from build123d import *

# Parameters (mm, degrees)
CYLINDER072_R     = 1.3
CYLINDER072_DEPTH = 331
CYLINDER061_R     = 1.3
CYLINDER061_DEPTH = 331
CYLINDER054_W     = 105
CYLINDER054_H     = 10
CYLINDER054_ANGLE = 180
CYLINDER053_W     = 115
CYLINDER053_H     = 10
CYLINDER053_ANGLE = 180


with BuildPart() as cilindro072:
    # Cylinder072 → Cylinder072 (new body)
    with BuildSketch(Plane(origin=(5, 224, 178), x_dir=(0, 0, -1), z_dir=(1, 0, 0))):
        Circle(CYLINDER072_R)
    extrude(amount=CYLINDER072_DEPTH)


with BuildPart() as cilindro061:
    # Cylinder061 → Cylinder061 (new body)
    with BuildSketch(Plane(origin=(5, 6, 178), x_dir=(0, 0, -1), z_dir=(1, 0, 0))):
        Circle(CYLINDER061_R)
    extrude(amount=CYLINDER061_DEPTH)


with BuildPart() as cilindro054:
    # Cylinder054 → Cylinder054 (revolve)
    with BuildSketch(Plane(origin=(-3, 115, 171), x_dir=(0, -1, 0), z_dir=(0, 0, -1))):
        with Locations((52.5, 5)):
            Rectangle(CYLINDER054_W, CYLINDER054_H)
    revolve(axis=Axis((-3, 115, 171), (-1, 0, 0)), revolution_arc=CYLINDER054_ANGLE)


with BuildPart() as cut081:
    # Cylinder053 → Cylinder053 (revolve)
    with BuildSketch(Plane(origin=(-3, 115, 171), x_dir=(0, -1, 0), z_dir=(0, 0, -1))):
        with Locations((57.5, 5)):
            Rectangle(CYLINDER053_W, CYLINDER053_H)
    revolve(axis=Axis((-3, 115, 171), (-1, 0, 0)), revolution_arc=CYLINDER053_ANGLE)

    # Cut067: cut Cilindro054
    add(cilindro054.part, mode=Mode.SUBTRACT)


with BuildPart() as cut081_1:
    # Cut067 placement: moved
    add(cut081.part.moved(Location((343, 0, -9))))

    # Cut072: cut Cilindro061
    add(cilindro061.part, mode=Mode.SUBTRACT)

    # Cut081: cut Cilindro072
    add(cilindro072.part, mode=Mode.SUBTRACT)


solid = cut081_1.part
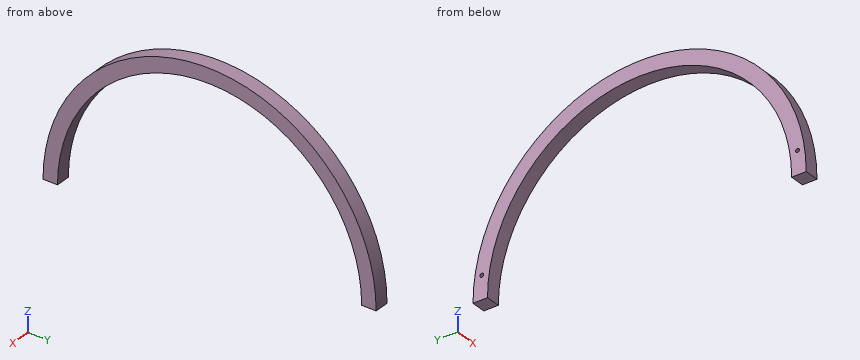
Design review of the part built by this model. Coordinates are the model's own, in mm. Give positions to 0.01 mm unless a question says otherwise; leave off trailing zeros. Order: outer loops, then holes, each group sorted by start corner. A loop starts at its lowest first (then second) coordinate and runs counter-clockwise, first axis right, second up. Notation, with made-up numbers: (25, 81) - (30, 81) arc R14 cw to (30, 105) - close; hole circle Ø6 at (85, -39). An arc over 180 degrees is marked (long way). Write item = value, one per line. Start each with the question number.
Q1. To check wall thickness, follow L1, parallel to Y at x = 333.25, z = 178; L2, parallel to Y at x = 338.5, z = 240; L3, parallel to Y at x = 337, z = 238. State the ranges of each line that lie inside material, in increasing order. Write a range as from..to.
Q2. We need section C-C on y = 115. State the section outline as (x, z) points.
Q3. We need section A-A on z = 195. State the section outline as (x, y) points, plus the area to 3 significant figures.
Q4. Clearance check with flat-ended pins moving along their axes: pin 1 Ø3 at (x, y) = (336.5, 56) entering from +Z; pin 2 Ø2 at (x, z) = (338, 196) entering from -Y; pin 3 Ø3.5 at (y, z) = (6, 178) entering from -X; pin 4 Ø4 at (x, y) = (331.5, 101) entering from +Z. State where each tip first meets the part, or that it passes through.
Q5. We need section B-B on x = 334.5. State the section outline as (y, z) points, plus the area to 3 significant figures.
Q6. We need section D-D on z = 242.5. State the section outline as (x, y) points.
Working result:
q1.L1 = 1.12..4.7, 7.3..11.23, 218.77..222.7, 225.3..228.88
q1.L2 = 30.5..44.71, 185.29..199.5
q1.L3 = 28.69..42.55, 187.45..201.31
q2.outline = (330, 267) - (340, 267) - (340, 277) - (330, 277) - close
q3.outline = (330, 4.84) - (340, 4.84) - (340, 15.32) - (330, 15.32) - close; (330, 214.68) - (340, 214.68) - (340, 225.16) - (330, 225.16) - close
q3.area = 210 mm²
q4.pin_1 = 261.59
q4.pin_2 = 4.84
q4.pin_3 = 330
q4.pin_4 = 276.37
q5.outline = (0, 162) - (10, 162) arc R105 cw to (220, 162) - (230, 162) arc R115 ccw to start; hole circle Ø2.6 at (6, 178); hole circle Ø2.6 at (224, 178)
q5.area = 3,450 mm²
q6.outline = (330, 32.87) - (340, 32.87) - (340, 47.59) - (330, 47.59) - close; (330, 182.41) - (340, 182.41) - (340, 197.13) - (330, 197.13) - close
